from build123d import *

# Parameters (mm, degrees)
F0_W      = 18.6
F0_H      = 3.6
F1_DEPTH  = 40
F2_W      = 1.5
F2_H      = 3.5
F3_DEPTH  = 40
F4_DEPTH  = 38
F5_DEPTH  = 11
F6_DEPTH  = 33
F2_H_2    = 8.25
F7_DEPTH  = 28
F8_R      = 3.86
F9_DEPTH  = 40000
F8_R_2    = 3.6
F10_DEPTH = 30


with BuildPart() as f1:
    # F0 (on Top) → F1 (new body)
    with BuildSketch(Plane.XY):
        with Locations((26.55, 11.8)):
            Rectangle(F0_W, F0_H)
        Polygon((17.25, 17.7), (-17.25, 17.7), (-17.25, -16.8), (17.25, -16.8), (17.25, -13.6), (17.25, -10), (17.25, 10), (17.25, 13.6), align=None)
        with Locations((26.55, -11.8)):
            Rectangle(F0_W, F0_H)
    extrude(amount=F1_DEPTH)

    # F2 (on face) → F3 (cut, through all)
    with BuildSketch(Plane(origin=(0, 0, 0), x_dir=(1, 0, 0), z_dir=(0, 0, -1))):
        with BuildLine():
            ThreePointArc((2.5, 0), (1.767766953, 1.767766953), (0, 2.5))
            Line((0, 2.5), (0, 1.75))
            Line((0, 1.75), (0, -1.75))
            Line((0, -1.75), (0, -2.5))
            ThreePointArc((0, -2.5), (1.767766953, -1.767766953), (2.5, 0))
        make_face()
        with BuildLine():
            Line((0, 1.75), (0, 2.5))
            ThreePointArc((0, 2.5), (-0.9682458366, 2.3048861143), (-1.7853571071, 1.75))
            Line((-1.7853571071, 1.75), (0, 1.75))
        make_face()
        with BuildLine():
            ThreePointArc((-1.7853571071, -1.75), (-0.9682458366, -2.3048861143), (0, -2.5))
            Line((0, -2.5), (0, -1.75))
            Line((0, -1.75), (-1.7853571071, -1.75))
        make_face()
        with BuildLine():
            Line((0, 1.75), (-1.7853571071, 1.75))
            ThreePointArc((-1.7853571071, 1.75), (-2.5, 0), (-1.7853571071, -1.75))
            Line((-1.7853571071, -1.75), (0, -1.75))
            Line((0, -1.75), (0, 1.75))
        make_face()
        with BuildLine():
            Line((-1.7853571071, 1.75), (-13.8901943831, 1.75))
            ThreePointArc((-13.8901943831, 1.75), (-14, 0), (-13.8901943831, -1.75))
            Line((-13.8901943831, -1.75), (-1.7853571071, -1.75))
            ThreePointArc((-1.7853571071, -1.75), (-2.5, 0), (-1.7853571071, 1.75))
        make_face()
        with BuildLine():
            ThreePointArc((-13.8901943831, -1.75), (-14, 0), (-13.8901943831, 1.75))
            Line((-13.8901943831, 1.75), (-15.75, 1.75))
            Line((-15.75, 1.75), (-15.75, -1.75))
            Line((-15.75, -1.75), (-13.8901943831, -1.75))
        make_face()
        with Locations((-16.5, 0)):
            Rectangle(F2_W, F2_H)
    extrude(amount=-F3_DEPTH, mode=Mode.SUBTRACT)

    # F2 (on face) → F4 (cut)
    with BuildSketch(Plane(origin=(0, 0, 0), x_dir=(1, 0, 0), z_dir=(0, 0, -1))):
        with BuildLine():
            ThreePointArc((-9.7979589711, -10), (3.1972216116, -13.6300320603), (13.2227077409, -4.6))
            Line((13.2227077409, -4.6), (0, -4.6))
            Line((0, -4.6), (0, -10))
            Line((0, -10), (-9.7979589711, -10))
        make_face()
        with BuildLine():
            Line((-1.7853571071, 1.75), (-13.8901943831, 1.75))
            ThreePointArc((-13.8901943831, 1.75), (-14, 0), (-13.8901943831, -1.75))
            Line((-13.8901943831, -1.75), (-1.7853571071, -1.75))
            ThreePointArc((-1.7853571071, -1.75), (-2.5, 0), (-1.7853571071, 1.75))
        make_face()
        with BuildLine():
            ThreePointArc((-13.8901943831, -1.75), (-12.5418410663, -6.2211110476), (-9.7979589711, -10))
            Line((-9.7979589711, -10), (0, -10))
            Line((0, -10), (0, -4.6))
            Line((0, -4.6), (0, -2.5))
            ThreePointArc((0, -2.5), (-0.9682458366, -2.3048861143), (-1.7853571071, -1.75))
            Line((-1.7853571071, -1.75), (-13.8901943831, -1.75))
        make_face()
        with BuildLine():
            Line((0, 10), (-9.7979589711, 10))
            ThreePointArc((-9.7979589711, 10), (-12.5418410663, 6.2211110476), (-13.8901943831, 1.75))
            Line((-13.8901943831, 1.75), (-1.7853571071, 1.75))
            ThreePointArc((-1.7853571071, 1.75), (-0.9682458366, 2.3048861143), (0, 2.5))
            Line((0, 2.5), (0, 4.6))
            Line((0, 4.6), (0, 10))
        make_face()
        with BuildLine():
            Line((0, 4.6), (13.2227077409, 4.6))
            ThreePointArc((13.2227077409, 4.6), (3.1972216116, 13.6300320603), (-9.7979589711, 10))
            Line((-9.7979589711, 10), (0, 10))
            Line((0, 10), (0, 4.6))
        make_face()
        with BuildLine():
            ThreePointArc((13.2227077409, -4.6), (13.8043092615, -2.3326049417), (14, 0))
            ThreePointArc((14, 0), (13.8043092615, 2.3326049417), (13.2227077409, 4.6))
            Line((13.2227077409, 4.6), (0, 4.6))
            Line((0, 4.6), (0, 2.5))
            ThreePointArc((0, 2.5), (1.767766953, 1.767766953), (2.5, 0))
            ThreePointArc((2.5, 0), (1.767766953, -1.767766953), (0, -2.5))
            Line((0, -2.5), (0, -4.6))
            Line((0, -4.6), (13.2227077409, -4.6))
        make_face()
    extrude(amount=-F4_DEPTH, mode=Mode.SUBTRACT)

    # F2 (on face) → F5 (cut)
    with BuildSketch(Plane(origin=(0, 0, 0), x_dir=(1, 0, 0), z_dir=(0, 0, -1))):
        with BuildLine():
            ThreePointArc((13.2227077409, 4.6), (13.8043092615, 2.3326049417), (14, 0))
            ThreePointArc((14, 0), (13.8043092615, -2.3326049417), (13.2227077409, -4.6))
            Line((13.2227077409, -4.6), (15.5454194173, -4.6))
            Line((15.5454194173, -4.6), (15.5454194173, 4.6))
            Line((15.5454194173, 4.6), (13.2227077409, 4.6))
        make_face()
    extrude(amount=-F5_DEPTH, mode=Mode.SUBTRACT)

    # F2 (on face) → F6 (cut)
    with BuildSketch(Plane(origin=(0, 0, 0), x_dir=(1, 0, 0), z_dir=(0, 0, -1))):
        with BuildLine():
            ThreePointArc((-13.8901943831, 1.75), (-12.5418410663, 6.2211110476), (-9.7979589711, 10))
            Line((-9.7979589711, 10), (-15.75, 10))
            Line((-15.75, 10), (-15.75, 1.75))
            Line((-15.75, 1.75), (-13.8901943831, 1.75))
        make_face()
        with BuildLine():
            ThreePointArc((-13.8901943831, -1.75), (-14, 0), (-13.8901943831, 1.75))
            Line((-13.8901943831, 1.75), (-15.75, 1.75))
            Line((-15.75, 1.75), (-15.75, -1.75))
            Line((-15.75, -1.75), (-13.8901943831, -1.75))
        make_face()
        with BuildLine():
            Line((-15.75, -10), (-9.7979589711, -10))
            ThreePointArc((-9.7979589711, -10), (-12.5418410663, -6.2211110476), (-13.8901943831, -1.75))
            Line((-13.8901943831, -1.75), (-15.75, -1.75))
            Line((-15.75, -1.75), (-15.75, -10))
        make_face()
    extrude(amount=-F6_DEPTH, mode=Mode.SUBTRACT)

    # F2 (on face) → F7 (cut)
    with BuildSketch(Plane(origin=(0, 0, 0), x_dir=(1, 0, 0), z_dir=(0, 0, -1))):
        with Locations((-16.5, 5.875)):
            Rectangle(F2_W, F2_H_2)
        with Locations((-16.5, -5.875)):
            Rectangle(F2_W, F2_H_2)
    extrude(amount=-F7_DEPTH, mode=Mode.SUBTRACT)

    # F8 (on face) → F9 (cut)
    with BuildSketch(Plane.XZ.offset(13.6)):
        with Locations((26.55, 8.547344245)):
            Circle(F8_R)
    extrude(amount=-F9_DEPTH, mode=Mode.SUBTRACT)

    # F8 (on face) → F10 (cut)
    with BuildSketch(Plane.XZ.offset(13.6)):
        with Locations((26.55, 22.8790044785)):
            Circle(F8_R_2)
    extrude(amount=-F10_DEPTH, mode=Mode.SUBTRACT)


solid = f1.part
Model file for the job. Use its own axes, mm. A direction names the side the tool comes from. Round coordinates to 2 decimals unless told otherwise and drop trailing zeros. Order: outer loops, then holes, each group sorted by start corner. A loop starts at its lowest first (then second) coordinate and runs counter-clockwise, first axis right, second up.
(1) Band-saw the part on B-B (x = 32). List the corners of the cut face in (y, z), then the cut area to 3 significant figures.
(2) Pull direction Y, two halves, no side cores. Call faces 5 (the face through (-17, 6, 28)), 6 (the face through (0, 17.7, 20)), 7 (the face through (22.694, -11.825, 8.717)): released by +Y, released by -Y, zero draft, split by the parting line, or undercut.
(3) Band-saw the part on D-D (z = 9.5). List the corners of the cut face in (x, y).
(4) 3-axis set-ups, long thin cutter, end or side, ignore diameter. For faces 1 (the face through (-14.1, -1.75, 36.2)), 2 (the face through (17.25, -15, 20)), 3 (the face through (-17, -6, 28)), 4 (the face through (35.85, -12, 20)): which of +Z, -Z, +X, -X, +Y, -Y reach the whole face in a straight line?
(5) Band-saw the part on C-C (z = 36.5). List the corners of the cut face in (x, y), then the cut area to 3 significant figures.
(6) Band-saw the part on A-A (x = 26.55). List the corners of the cut face in (y, z).
(7) Drill centre lines: line 1 (Z direction, x = 26.55, y = 11.55); line 2 (Y direction, x = 31.5, z = 28.5); line 3 (X direction, y = -3, z = 10). Where is each one in solid material? Low to high.
(8) Pin check, flat tips, straight feed: pin 1 (0.7 mm diameter, centred on x = 14.5, y = -1.5, fed in from -Z); pin 2 (0.8 mm diameter, centred on x = -16.5, y = 5, fed in from -Z); pin 3 (10 mm diameter, centred on x = 10.5, y = 4, fed in from -Z); pin 4 (2 mm diameter, centred on y = 15, z = 23.5, fed in from +X). Stop position of each tip, or through.
Verdict:
1. outline: (-13.6, 0) - (-10, 0) - (-10, 40) - (-13.6, 40) - close; (10, 0) - (13.6, 0) - (13.6, 40) - (10, 40) - close
1. area: 288 mm2
2. face 5: undercut
2. face 6: released by +Y
2. face 7: zero draft
3. outline: (-17.25, -16.8) - (17.25, -16.8) - (17.25, -13.6) - (22.81, -13.6) - (22.81, -10) - (17.25, -10) - (17.25, 10) - (22.81, 10) - (22.81, 13.6) - (17.25, 13.6) - (17.25, 17.7) - (-17.25, 17.7) - (-17.25, 10) - (-9.8, 10) arc R14 cw to (13.22, 4.6) - (15.55, 4.6) - (15.55, -4.6) - (13.22, -4.6) arc R14 cw to (-9.8, -10) - (-17.25, -10) - close; (30.29, -13.6) - (35.85, -13.6) - (35.85, -10) - (30.29, -10) - close; (30.29, 10) - (35.85, 10) - (35.85, 13.6) - (30.29, 13.6) - close
4. face 1: +Z, -Z, -X
4. face 2: +Z, -Z, +X, -Y
4. face 3: -Z, -X
4. face 4: +Z, -Z, +X, +Y, -Y
5. outline: (-17.25, -16.8) - (17.25, -16.8) - (17.25, -13.6) - (35.85, -13.6) - (35.85, -10) - (17.25, -10) - (17.25, 10) - (35.85, 10) - (35.85, 13.6) - (17.25, 13.6) - (17.25, 17.7) - (-17.25, 17.7) - (-17.25, 1.75) - (-13.89, 1.75) arc R14 cw (long way) to (-13.89, -1.75) - (-17.25, -1.75) - close
5. area: 697 mm2
6. outline: (-13.6, 0) - (-10, 0) - (-10, 4.69) - (-13.6, 4.69) - close; (-13.6, 12.41) - (-10, 12.41) - (-10, 19.28) - (-13.6, 19.28) - close; (-13.6, 26.48) - (-10, 26.48) - (-10, 40) - (-13.6, 40) - close; (10, 0) - (13.6, 0) - (13.6, 4.69) - (10, 4.69) - close; (10, 12.41) - (13.6, 12.41) - (13.6, 19.28) - (10, 19.28) - close; (10, 26.48) - (13.6, 26.48) - (13.6, 40) - (10, 40) - close
7. line 1: z = 0 to 4.69, 12.41 to 19.28, 26.48 to 40
7. line 2: y = -13.6 to -10, 10 to 13.6
7. line 3: x = 15.55 to 17.25
8. pin 1: stops at z = 11
8. pin 2: stops at z = 28
8. pin 3: stops at z = 0
8. pin 4: stops at x = 17.25
